Autodesk Inventor part; units mm, degrees
ref_plane "Arbeitsebene1" through (19, 0, 0) normal (1, 0, 0) x (0, 1, 0)
ref_plane "XZ Plane" through (0, 0, 0) normal (0, 1, 0) x (-1, 0, 0)
ref_plane "XY Plane" through (0, 0, 0) normal (0, 0, 1) x (1, 0, 0)
sketch "Skizze1" plane through (0, 0, 0) normal (0, 1, 0) x (-1, 0, 0)
  line L0 (14, 0) -> (-14, 0) construction
  line L1 (14, -5) -> (-14, -5)
  line L2 (-14, 5) -> (14, 5)
  arc A0 (14, -5) -> (14, 5) centre (14, 0) ccw
  arc A1 (-14, 5) -> (-14, -5) centre (-14, 0) ccw
  point P0 (0, 0)
  point P1 (0, 0)
  point P2 (-19, 0)
  point P3 (19, 0)
  dimension "d1" = 38
  dimension "d2" = 5
extrude "Extrusion1" add sketch "Skizze1" along normal blind 10
sketch "Skizze2" plane through (0, 10, 0) normal (0, 1, 0) x (1, 0, 0)
  point P0 (0, 0)
  point P1 (0, 0)
hole "Bohrung1" at (0, 10, 0) direction (0, -1, 0) diameter 6.5 depth 10
sketch "Skizze3" plane through (0, 10, 0) normal (0, 1, 0) x (1, 0, 0)
  point P0 (0, 0)
  point P1 (-12.5, 0)
  dimension "d19" = 12.5
hole "Bohrung2" at (-12.5, 10, 0) direction (0, -1, 0) diameter 4 end through all
ref_plane "Arbeitsebene1" through (19, 0, 0) normal (1, 0, 0) x (0, 1, 0)
sketch "Skizze4" plane through (19, 0, 0) normal (1, 0, 0) x (0, 1, 0)
  line L0 (0, -5) -> (0, 5)
  point P0 (0, 0)
  point P1 (5, 0)
  point P2 (0, 0)
  dimension "d21" = 5
hole "Bohrung3" at (19, 5, 0) direction (-1, 0, 0) diameter 3.242 depth 15.75 tip angle 118
properties part number "BMS_small" material "Gummi"
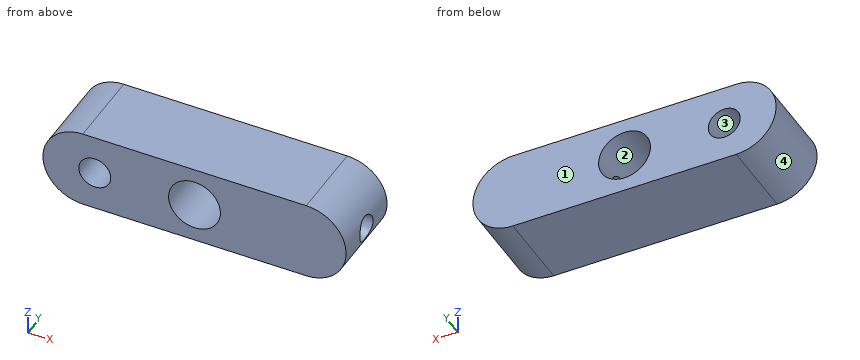
The model under review builds one solid part; all positions refer to its coordinate system, in mm. Face numbers are marked on the shaded views. Round coordinates to 2 decimals unless told otherwise and drop trailing zeros. Write each loop counter-clockwise with the first axis right and the second up, starting at its lowest first coordinate (ties: lowest second). Pieces come first, ordered by that corner, then holes. Notation, with made-up numbers: (2.25, -11.75) -> (8.25, -11.75) arc R16 ccw to (8.25, 16.25) -> close; hole circle Ø5 at (-24, 42). An arc over 180 degrees is marked (long way). Use CSV: the item, a comma, the result in double quotes.
Q1. Consider section B-B (y = 1.75). Give the boundary of the cut face in (x, z), then the cut area to 3 significant figures.
Checks:
outline,"(-14, -5) -> (14, -5) arc R5 ccw to (14, 5) -> (-14, 5) arc R5 ccw to start; hole circle Ø4 at (-12.5, 0); hole circle Ø6.5 at (0, 0)"
area,"313 mm²"
Q2. Consider section A-A (x = 0). Give the boundary of the cut face in (y, z), then the cut area to 3 significant figures.
Checks:
outline,"(0, -5) -> (10, -5) -> (10, -3.25) -> (0, -3.25) -> close; (0, 3.25) -> (10, 3.25) -> (10, 5) -> (0, 5) -> close"
area,"35.0 mm²"
Q3. Mouldability with a two-part tool opening along X and no side actions: class the marked faces 1, 2, 3 and 4 as released by +X, released by -X, zero draft, split by the parting line, or undercut.
Checks:
face 1,"zero draft"
face 2,"undercut"
face 3,"undercut"
face 4,"released by -X"
Q4. To check wall thickness, follow probe 1 along Z at (x, y) = (0, 4); probe 2 along X at (y, z) = (6.75, 0); probe 3 along X at (y, z) = (7, -0.5). State the ranges of each line that lie inside material, in increasing order. Write a range as [from, to].
Checks:
probe 1,"[-5, -3.25], [3.25, 5]"
probe 2,"[-19, -14.5], [-10.5, -3.25], [3.25, 19]"
probe 3,"[-18.97, -14.44], [-10.56, -3.21], [3.21, 18.97]"
Q5. Consider section C-C (y = 5). Give the boundary of the cut face in (x, z), then the cut area to 3 significant figures.
Checks:
outline,"(-14, -5) -> (14, -5) arc R5 ccw to (18.73, -1.62) -> (3.25, -1.62) -> (3.01, -1.22) arc R3.25 cw (long way) to (3.01, 1.22) -> (3.25, 1.62) -> (18.73, 1.62) arc R5 ccw to (14, 5) -> (-14, 5) arc R5 ccw to start; hole circle Ø4 at (-12.5, 0)"
area,"262 mm²"
Q6. For pin 1 Ø1 at (y, z) = (8.5, -2.5) entering from +X, flat-tipped, find the tip position at first contact; note if it passes through.
Checks:
pin 1,"x = 18.58"
Q7. Consider section D-D (z = -2.75). Give the boundary of the cut face in (x, y), then the cut area to 3 significant figures.
Checks:
outline,"(-18.18, 0) -> (-1.73, 0) -> (-1.73, 10) -> (-18.18, 10) -> close; (1.73, 0) -> (18.18, 0) -> (18.18, 10) -> (1.73, 10) -> close"
area,"329 mm²"
